```python
from build123d import *

# Parameters (mm, degrees)
SKETCH1_R           = 30
SKETCH1_R_2         = 2.5
BOSS_EXTRUDE1_DEPTH = 5
SKETCH2_R           = 5
BOSS_EXTRUDE2_DEPTH = 75
FILLET1_R           = 2.5


with BuildPart() as part:
    # Sketch1 → Boss-Extrude1 (new body)
    with BuildSketch(Plane(origin=(0, 0, 0), x_dir=(1, 0, 0), z_dir=(0, 1, 0))):
        with Locations(Location((0, 0, 0), (0, 0, 270))):
            Circle(SKETCH1_R)
        with Locations(Location((-20.56810334, 11.875, 0), (0, 0, 270))):
            Circle(SKETCH1_R_2, mode=Mode.SUBTRACT)
        with Locations(Location((0, 23.75, 0), (0, 0, 270))):
            Circle(SKETCH1_R_2, mode=Mode.SUBTRACT)
        with Locations(Location((20.56810334, 11.875, 0), (0, 0, 270))):
            Circle(SKETCH1_R_2, mode=Mode.SUBTRACT)
        with Locations(Location((20.56810334, -11.875, 0), (0, 0, 270))):
            Circle(SKETCH1_R_2, mode=Mode.SUBTRACT)
        with Locations(Location((0, -23.75, 0), (0, 0, 270))):
            Circle(SKETCH1_R_2, mode=Mode.SUBTRACT)
        with Locations(Location((-20.56810334, -11.875, 0), (0, 0, 270))):
            Circle(SKETCH1_R_2, mode=Mode.SUBTRACT)
    extrude(amount=BOSS_EXTRUDE1_DEPTH)

    # Sketch2 → Boss-Extrude2 (add)
    with BuildSketch(Plane(origin=(0, 5, 0), x_dir=(1, 0, 0), z_dir=(0, 1, 0))):
        with Locations(Location((0, 0, 0), (0, 0, 270))):
            Circle(SKETCH2_R)
    extrude(amount=BOSS_EXTRUDE2_DEPTH)

    # Fillet1
    fillet1_edges = [part.edges().sort_by_distance(p)[0] for p in [
        (0, 5, -5),
    ]]
    fillet(fillet1_edges, radius=FILLET1_R)


solid = part.part
```
The listing builds one solid part. Answer for the finished solid, in the listing's coordinates (mm). A direction names the side the tool comes from. Give positions to 0.01 mm unless a question says otherwise; leave off trailing zeros. Order: outer loops, then holes, each group sorted by start corner. A loop starts at its lowest first (then second) coordinate and runs counter-clockwise, first axis right, second up. Notation, with made-up numbers: (4, 74.5) -> (45, 74.5) arc R17 ccw to (45, 93.5) -> close; hole circle Ø8 at (-3.75, 21). An arc over 180 degrees is marked (long way). One line per item, written item: value.
1) A tool of negligible diameter and unlimited length cuts with its end or side. For faces 1 (the cylindrical face through (0.11, 2.465, 21.252)), 2 (the flat face through (-6, 5, 6)), from which of +Z, -Z, +X, -X, +Y, -Y can it reach the whole face along a straight path? Write none if from no direction.
Reported:
face 1: +Y, -Y
face 2: +Y
2) Determine the mould class of faces 3 (the flat face through (0, 0, 0)), 4 (the cylindrical face through (23.047, 2.465, 11.55)), 5 (the cylindrical face through (23.047, 2.465, -12.2)), 6 (the cylindrical face through (-4.88, 43.24, -1.08)) for opening direction Z: pulls with the +Z half, pulls with the -Z half, needs draft (parallel to the pull), parting line crosses it, or undercut.
Reported:
face 3: needs draft
face 4: undercut
face 5: undercut
face 6: parting line crosses it
3) Find section B-B, the plane z = -23.75. Determine the outline of the cut face in (x, y).
Reported:
outline: (-18.33, 0) -> (-2.5, 0) -> (-2.5, 5) -> (-18.33, 5) -> close; (2.5, 0) -> (18.33, 0) -> (18.33, 5) -> (2.5, 5) -> close
4) Find section C-C, the plane z = 0. Determine the outline of the cut face in (x, y).
Reported:
outline: (-30, 0) -> (30, 0) -> (30, 5) -> (7.5, 5) arc R2.5 cw to (5, 7.5) -> (5, 80) -> (-5, 80) -> (-5, 7.5) arc R2.5 cw to (-7.5, 5) -> (-30, 5) -> close
5) Flat-ended cylindrical pins translate along their axes: P1, Ø8, axis at x = -20.57, z = -11.88, coming from the +Y side; P2, Ø1.5, axis at y = 48, z = -6.5, coming from the -X side; P3, Ø8, axis at x = -20.57, z = 11.88, coming from the -Y side; P4, Ø12, axis at x = -11.5, z = 0, coming from the +Y side. Find the tip coordinate at first contact, or state that the pin passes through.
Reported:
P1: stops at y = 5
P2: passes through
P3: stops at y = 0
P4: stops at y = 6
6) Find section D-D, the plane y = 18. Determine the outline of the cut face in (x, z), plus the area to 3 significant figures.
Reported:
outline: circle Ø10 at (0, 0)
area: 78.5 mm^2
7) Find the intervals of material crossed by line 1 (Y direction, x = -12, z = 22); line 2 (Z direction, x = 1, y = 33.5); line 3 (X direction, y = 1, z = -23), in increasing order.
Reported:
line 1: y = 0 to 5
line 2: z = -4.9 to 4.9
line 3: x = -19.26 to -2.38, 2.38 to 19.26
8) Find section A-A, the plane x = 0. Determine the outline of the cut face in (y, z).
Reported:
outline: (0, -30) -> (5, -30) -> (5, -26.25) -> (0, -26.25) -> close; (0, -21.25) -> (5, -21.25) -> (5, -7.5) arc R2.5 cw to (7.5, -5) -> (80, -5) -> (80, 5) -> (7.5, 5) arc R2.5 cw to (5, 7.5) -> (5, 21.25) -> (0, 21.25) -> close; (0, 26.25) -> (5, 26.25) -> (5, 30) -> (0, 30) -> close
